Design review of the part built by this model. Coordinates are the model's own, in mm. Face numbers are marked on the shaded views. A direction names the side the tool comes from. Give positions to 0.01 mm unless a question says otherwise; leave off trailing zeros. Order: outer loops, then holes, each group sorted by start corner. A loop starts at its lowest first (then second) coordinate and runs counter-clockwise, first axis right, second up. Notation, with made-up numbers: (51, 52) -> (76, 52) arc R27 cw to (76, 80) -> close; hole circle Ø10 at (76.25, 45). An arc over 180 degrees is marked (long way). One line per item, written item: value. Start each with the question number.
1) Consider section C-C (y = 3.5). State the section outline as (x, z) points.
2) Consider section A-A (z = 0). State the section outline as (x, y) points, plus the area to 3 significant figures.
3) The part is to be moulded in two halves that separate along Z. For the marked faces 4, 5 and 6, say which applies: released by +Z, released by -Z, zero draft, split by the parting line, or undercut.
4) Tool access review of the marked faces 1, 2 and 3: name each direction out of +Z, -Z, +X, -X, +Y, -Y from which nothing blocks a thin tool from reaching the whole face with its end or side.
5) Consider section D-D (x = 0.35). State the section outline as (y, z) points, plus the area to 3 significant figures.
6) Wall thickness on line 1 along Z through (x, y) = (0.05, 7.25); line 2 along Y through (x, z) = (0.1, 2.4); line 3 along Y through (x, z) = (0.35, 0.65): over which ranges is each line inside the solid? List them lowest first. Write a range as from..to.
7) For pin 1 (1 mm diameter, centred on x = 0, z = 0.5, fed in from -Y); pin 2 (3 mm diameter, centred on x = -0.5, y = 6, fed in from -Z); pin 3 (1 mm diameter, centred on x = 1.5, y = 6, fed in from +Z), all flat-tipped, find the tip position at first contact; note any pin that passes through.
8) Consider section B-B (x = -1.3). State the section outline as (y, z) points, plus the area to 3 significant figures.
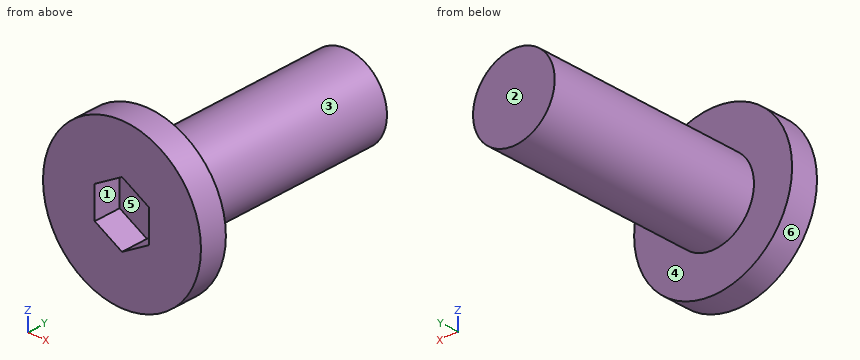
Autodesk Inventor part; units mm, degrees
ref_plane "YZ Plane" through (0, 0, 0) normal (1, 0, 0) x (0, 1, 0)
ref_plane "XZ Plane" through (0, 0, 0) normal (0, 1, 0) x (-1, 0, 0)
ref_plane "XY Plane" through (0, 0, 0) normal (0, 0, 1) x (1, 0, 0)
sketch "Sketch1" plane through (0, 0, 0) normal (0, 1, 0) x (-1, 0, 0)
  circle A0 centre (0, 0) radius 2.9
  dimension "d0" = 5.8
extrude "Extrusion1" add sketch "Sketch1" along normal blind 1
sketch "Sketch2" plane through (0, 1, 0) normal (0, 1, 0) x (1, 0, 0)
  circle A0 centre (0, 0) radius 1.5
  dimension "d3" = 3
extrude "Extrusion2" add sketch "Sketch2" along normal blind 8
sketch "Sketch3" plane through (0, 0, 0) normal (0, -1, 0) x (1, 0, 0)
  line L0 (0, -1.1547) -> (-1, -0.5774)
  line L1 (-1, -0.5774) -> (-1, 0.5774)
  line L2 (-1, 0.5774) -> (0, 1.1547)
  line L3 (0, 1.1547) -> (1, 0.5774)
  line L4 (1, 0.5774) -> (1, -0.5774)
  line L5 (1, -0.5774) -> (0, -1.1547)
  point P0 (0, 0)
  point P1 (0, 0)
  dimension "d6" = 2
extrude "Extrusion3" cut sketch "Sketch3" against normal blind 1
properties part number "m3_bolt_pan_8mm" material "Stainless Steel"
Checked values:
1. outline: circle Ø3 at (0, 0)
2. outline: (-2.9, 0) -> (-1, 0) -> (-1, 1) -> (1, 1) -> (1, 0) -> (2.9, 0) -> (2.9, 1) -> (1.5, 1) -> (1.5, 9) -> (-1.5, 9) -> (-1.5, 1) -> (-2.9, 1) -> close
2. area: 27.8 mm^2
3. face 4: zero draft
3. face 5: undercut
3. face 6: split by the parting line
4. face 1: -Y
4. face 2: +Z, -Z, +X, -X, +Y
4. face 3: +Y
5. outline: (0, -2.88) -> (1, -2.88) -> (1, -1.46) -> (9, -1.46) -> (9, 1.46) -> (1, 1.46) -> (1, 2.88) -> (0, 2.88) -> (0, 0.95) -> (1, 0.95) -> (1, -0.95) -> (0, -0.95) -> close
5. area: 27.2 mm^2
6. line 1: z = -1.5..1.5
6. line 2: y = 0..1
6. line 3: y = 1..9
7. pin 1: stops at y = 1
7. pin 2: stops at z = -1.5
7. pin 3: stops at z = 1.12
8. outline: (0, -2.59) -> (1, -2.59) -> (1, -0.75) -> (9, -0.75) -> (9, 0.75) -> (1, 0.75) -> (1, 2.59) -> (0, 2.59) -> close
8. area: 17.2 mm^2
